CAD build for the part. Positions are in the model's coordinates, mm. A direction names the side the tool comes from. Coordinates: 2 decimals unless noted, no trailing zeros. Order: outer loops, then holes, each group sorted by start corner. A loop starts at its lowest first (then second) coordinate and runs counter-clockwise, first axis right, second up. Notation, with made-up numbers: M 85.25,45.25 L 140.25,45.25 A31 cw 140.25,74.25 Z; hole C 73,26 d10. An arc over 180 degrees is marked long. Write item = value, one per line. Start each with the question number.
```python
from build123d import *

# Parameters (mm, degrees)
F0_R     = 9
F1_DEPTH = 3
F3_DEPTH = 3
F4_R     = 1.75
F5_DEPTH = 3
F7_SIZE  = 1


# Not quite as in the source:
# - a feature names something its author has since deleted; it is built from what else it names


with BuildPart() as f1:
    # F0 (on Top) → F1 (new body)
    with BuildSketch(Plane.XY):
        with BuildLine():
            Line((55.375, -31.75), (55.375, 31.75))
            Line((55.375, 31.75), (0, 31.75))
            ThreePointArc((0, 31.75), (-31.75, 0), (0, -31.75))
            Line((0, -31.75), (55.375, -31.75))
        make_face()
        Circle(F0_R, mode=Mode.SUBTRACT)
    extrude(amount=F1_DEPTH)

    # F2 (on face) → F3 (join)
    with BuildSketch(Plane(origin=(0, 0, 0), x_dir=(1, 0, 0), z_dir=(0, 0, -1))):
        with BuildLine():
            ThreePointArc((0, 31.75), (-31.75, 0), (0, -31.75))
            Line((0, -31.75), (55.375, -31.75))
            Line((55.375, -31.75), (55.375, 31.75))
            Line((55.375, 31.75), (0, 31.75))
        make_face()
        with BuildLine():
            Line((52.375, -28.75), (0, -28.75))
            ThreePointArc((0, -28.75), (-28.75, 0), (0, 28.75))
            Line((0, 28.75), (52.375, 28.75))
            Line((52.375, 28.75), (52.375, -28.75))
        make_face(mode=Mode.SUBTRACT)
    extrude(amount=F3_DEPTH)

    # F4 (on face) → F5 (join)
    with BuildSketch(Plane.XZ.offset(31.75)):
        with BuildLine():
            Line((14.75, -3), (2.75, -3))
            Line((2.75, -3), (2.75, -10))
            ThreePointArc((2.75, -10), (8.75, -16), (14.75, -10))
            Line((14.75, -10), (14.75, -3))
        make_face()
        with Locations((8.75, -10)):
            Circle(F4_R, mode=Mode.SUBTRACT)
    extrude(amount=-F5_DEPTH)

    # F6: F1 across plane


with BuildPart() as f1_1:
    add(f1.part)
    add(f1.part.mirror(Plane.XZ))

    # F7
    f7_edges = [f1_1.edges().sort_by_distance(p)[0] for p in [
        (7, -31.75, -10),
        (7, 31.75, -10),
    ]]
    chamfer(f7_edges, length=F7_SIZE)


solid = f1_1.part
```
1. Flat gauge pins, fed straight in: pin 1 (10 mm diameter, centred on y = -1.5, z = -3, fed in from -X); pin 2 (3.5 mm diameter, centred on y = 30, z = -7.5, fed in from +X); pin 3 (8 mm diameter, centred on x = -16, z = -5, fed in from -Y). Where does each tip first touch, or does it go through?
2. Probe L1, parallel to Z at x = 8.75, y = 30; L2, parallel to Y at x = 28, z = -1; L3, parallel to Y at x = 0, z = 1. List the from-to ranges inside material, lowest first.
3. Slice it at A-A (y = 0). Write the cut outline in (x, z) (3 decimals), plus the area to 3 significant figures.
4. 3-axis set-ups, long thin cutter, end or side, ignore diameter. For faces 5 (the flat face through (14.75, 30, -7)), 6 (the flat face through (55.375, 0, 0)), 7 (the flat face through (22, -31.75, -2)), 8 (the flat face through (-29, -5, -3)), 9 (the flat face through (11, 0, 0)): which of +Z, -Z, +X, -X, +Y, -Y reach the whole face in a straight line?
5. Mould opens along Z. For faces 1 (the cylindrical face through (9.691, -29.764, -8.524)), 2 (the cylindrical face through (9.691, 29.764, -8.524)), 3 (the flat face through (52.375, 0, -1)), 4 (the flat face through (11, 0, 3)) say: released by +Z, released by -Z, zero draft, split by the parting line, or undercut.
6. Slice it at C-C (z = -1.25). Write the cut outline in (x, y) (3 decimals), plus the area to 3 significant figures.
7. Slice it at D-D (x = 23.5). Write the cut outline in (y, z), plus the area to 4 significant figures.
8. Slice it at B-B (z = -5.25). Write the cut outline in (x, y).
Calculated:
q1.pin_1 = -31.75
q1.pin_2 = 14.75
q1.pin_3 = -29.17
q2.L1 = -16 to -11.75, -8.25 to 3
q2.L2 = -31.75 to -28.75, 28.75 to 31.75
q2.L3 = -31.75 to -9, 9 to 31.75
q3.outline = M -31.75,-3 L -28.75,-3 L -28.75,0 L -9,0 L -9,3 L -31.75,3 Z; M 9,0 L 52.375,0 L 52.375,-3 L 55.375,-3 L 55.375,3 L 9,3 Z
q3.area = 225 mm²
q4.face_5 = -Z, +X, +Y, -Y
q4.face_6 = +Z, -Z, +X, +Y, -Y
q4.face_7 = +Z, -Z, +X, -X, -Y
q4.face_8 = -Z, -X, +Y, -Y
q4.face_9 = -Z
q5.face_1 = undercut
q5.face_2 = undercut
q5.face_3 = zero draft
q5.face_4 = released by +Z
q6.outline = M 0,-31.75 L 55.375,-31.75 L 55.375,31.75 L 0,31.75 A31.75 ccw Z; hole M 0,-28.75 L 52.375,-28.75 L 52.375,28.75 L 0,28.75 A28.75 ccw Z
q6.area = 790 mm²
q7.outline = M -31.75,-3 L -28.75,-3 L -28.75,0 L 28.75,0 L 28.75,-3 L 31.75,-3 L 31.75,3 L -31.75,3 Z
q7.area = 208.5 mm²
q8.outline = M 2.75,-31.75 L 14.75,-31.75 L 14.75,-28.75 L 2.75,-28.75 Z; M 2.75,28.75 L 14.75,28.75 L 14.75,31.75 L 2.75,31.75 Z
